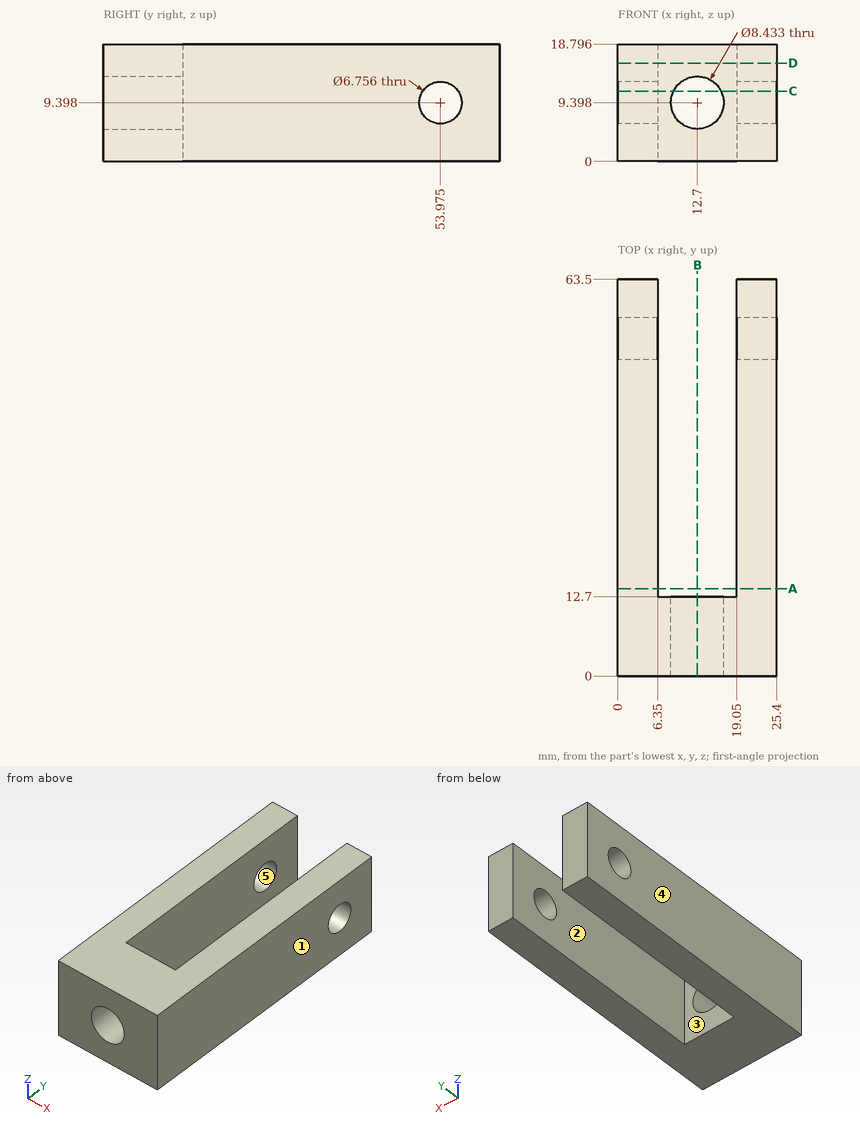
Drawing for the job (mm, zero at the part's lowest x, y, z). A direction names the side the tool comes from. Give positions to 0.01 mm unless a question says otherwise; leave off trailing zeros. Loops run counter-clockwise (first coordinate to the right, second up) from the corner with the lowest first, then second, coordinate; pieces in that order, holes last.
(1) Band-saw the part on D-D (z = 15.75). Write the cut outline in (x, y).
Return value:
outline: (0, 0) - (25.4, 0) - (25.4, 63.5) - (19.05, 63.5) - (19.05, 12.7) - (6.35, 12.7) - (6.35, 63.5) - (0, 63.5) - close
(2) Pin check, flat tips, straight feed: pin 1 (5 mm diameter, centred on x = 19, y = 19.5, fed in from -Z); pin 2 (10 mm diameter, centred on x = 12.5, z = 7, fed in from +Y). Stop position of each tip, or through.
Return value:
pin 1: stops at z = 0
pin 2: stops at y = 12.7
(3) Band-saw the part on B-B (x = 12.7). Write the cut outline in (y, z) (1 decimal).
Return value:
outline: (0, 0) - (12.7, 0) - (12.7, 5.2) - (0, 5.2) - close; (0, 13.6) - (12.7, 13.6) - (12.7, 18.8) - (0, 18.8) - close
(4) Drill centre lines: line 1 along X through (y, z) = (34, 8); line 2 along Y through (x, z) = (18.5, 4); line 3 along Y through (x, z) = (22.5, 9). Where is each one in solid material? Low to high.
Return value:
line 1: x = 0 to 6.35, 19.05 to 25.4
line 2: y = 0 to 12.7
line 3: y = 0 to 50.62, 57.33 to 63.5
(5) 3-axis set-ups, long thin cutter, end or side, ignore diameter. For the marked faces 1 and 2: which of +Z, -Z, +X, -X, +Y, -Y reach the whole face in a straight line?
Return value:
face 1: +Z, -Z, +X, +Y, -Y
face 2: +Z, -Z, +Y
(6) Band-saw the part on C-C (z = 11.25). Write the cut outline in (x, y).
Return value:
outline: (0, 0) - (8.91, 0) - (8.91, 12.7) - (6.35, 12.7) - (6.35, 51.15) - (0, 51.15) - close; (0, 56.8) - (6.35, 56.8) - (6.35, 63.5) - (0, 63.5) - close; (16.49, 0) - (25.4, 0) - (25.4, 51.15) - (19.05, 51.15) - (19.05, 12.7) - (16.49, 12.7) - close; (19.05, 56.8) - (25.4, 56.8) - (25.4, 63.5) - (19.05, 63.5) - close
(7) Pull direction Y, two halves, no side cores. Call the marked faces 3, 4 and 5: pulls with the +Y half, pulls with the -Y half, needs draft (parallel to the pull), parting line crosses it, or undercut.
Return value:
face 3: pulls with the +Y half
face 4: needs draft
face 5: undercut
(8) Band-saw the part on A-A (y = 14). Write the cut outline in (x, z), and give its area (3 significant figures).
Return value:
outline: (0, 0) - (6.35, 0) - (6.35, 18.8) - (0, 18.8) - close; (19.05, 0) - (25.4, 0) - (25.4, 18.8) - (19.05, 18.8) - close
area: 239 mm2
